from build123d import *

# Parameters (mm, degrees)
F0_R     = 13
F0_R_2   = 11.3
F0_R_3   = 7.4
F0_R_4   = 5
F1_DEPTH = 8
F2_DEPTH = 0.5
F3_START = 7.5
F3_DEPTH = 0.5
F4_SIZE  = 0.15


with BuildPart() as f1:
    # F0 (on Top) → F1 (new body)
    with BuildSketch(Plane.XY):
        Circle(F0_R)
        Circle(F0_R_2, mode=Mode.SUBTRACT)
        Circle(F0_R_2)
        Circle(F0_R_3, mode=Mode.SUBTRACT)
        Circle(F0_R_3)
        Circle(F0_R_4, mode=Mode.SUBTRACT)
    extrude(amount=F1_DEPTH)

    # F0 (on Top) → F2 (cut)
    with BuildSketch(Plane.XY):
        Circle(F0_R_2)
        Circle(F0_R_3, mode=Mode.SUBTRACT)
    extrude(amount=F2_DEPTH, mode=Mode.SUBTRACT)

    # F0 (on Top) → F3 (cut)
    with BuildSketch(Plane.XY.offset(F3_START)):
        Circle(F0_R_2)
        Circle(F0_R_3, mode=Mode.SUBTRACT)
    extrude(amount=F3_DEPTH, mode=Mode.SUBTRACT)

    # F4
    f4_edges = [f1.edges().sort_by_distance(p)[0] for p in [
        (-13, 0, 0),
        (-11.3, 0, 0),
        (-7.4, 0, 0),
        (-5, 0, 0),
        (-13, 0, 8),
        (-11.3, 0, 8),
        (-7.4, 0, 8),
        (-5, 0, 8),
    ]]
    chamfer(f4_edges, length=F4_SIZE)


solid = f1.part
The model under review builds one solid part; all positions refer to its coordinate system, in mm. A direction names the side the tool comes from. Coordinates: 2 decimals unless noted, no trailing zeros. Write each loop counter-clockwise with the first axis right and the second up, starting at its lowest first coordinate (ties: lowest second). Pieces come first, ordered by that corner, then holes. Notation, with made-up numbers: (53.5, 55.25) -> (92.5, 55.25) arc R26 ccw to (92.5, 71.25) -> close; hole circle Ø4 at (43.25, 28). An arc over 180 degrees is marked (long way). Answer in a Markdown table with one row per item.
1. We need section A-A, the plane z = 2.25. State the section outline as (x, y) points.
Answers below:
| item | result |
|---|---|
| outline | circle Ø26 at (0, 0); hole circle Ø10 at (0, 0) |
2. Wall thickness on probe 1 along Y at (x, z) = (0, 7.65); probe 2 along Y at (x, z) = (0, 3.25); probe 3 along Z at (x, y) = (-9, 4): over which ranges is each line inside the solid? List them lowest first. Write a range as [from, to].
Answers below:
| item | result |
|---|---|
| probe 1 | y = [-13, -11.3], [-7.4, -5], [5, 7.4], [11.3, 13] |
| probe 2 | y = [-13, -5], [5, 13] |
| probe 3 | z = [0.5, 7.5] |
3. Clearance check with flat-ended pins moving along their axes: pin 1 Ø4 at (y, z) = (-5.5, 4.5) entering from +X; pin 2 Ø1.5 at (x, y) = (-8, 1) entering from -Z; pin 3 Ø1 at (x, z) = (-9.5, 4.5) entering from -Y. State where each tip first meets the part, or that it passes through.
Answers below:
| item | result |
|---|---|
| pin 1 | stops at x = 12.52 |
| pin 2 | stops at z = 0.06 |
| pin 3 | stops at y = -9.38 |
4. For faces 1 (the flat face through (2, 5, 8)), 2 (the cylindrical face through (-1.604, -7.224, 7.673)), 3 (the cylindrical face through (-1.604, -7.224, 0.323)), list the 3-axis set-ups (+Z, -Z, +X, -X, +Y, -Y) from which the entire face can be reached by the end or side of a thin tool; tool diameter is ignored.
Answers below:
| item | result |
|---|---|
| face 1 | +Z, +X, -X, +Y, -Y |
| face 2 | +Z |
| face 3 | -Z |
5. Draft analysis for pull direction Y (two halves, no side actions). For faces 4 (the flat face through (2, 5, 0)), 5 (the cylindrical face through (-10.316, -7.91, 3.946)), 6 (the flat face through (7.4, -2.4, 7.5)), state which applies: +Y half, -Y half, draft (parallel to the pull), parting line (faces both ways), or undercut.
Answers below:
| item | result |
|---|---|
| face 4 | draft |
| face 5 | parting line |
| face 6 | undercut |
